Check sheet for the modelled part. Datum: model origin and axes. Units: mm. Face numbers are marked on the shaded views. A direction names the side the tool comes from. Give positions to 0.01 mm unless a question says otherwise; leave off trailing zeros. Write each loop counter-clockwise with the first axis right and the second up, starting at its lowest first coordinate (ties: lowest second). Pieces come first, ordered by that corner, then holes.
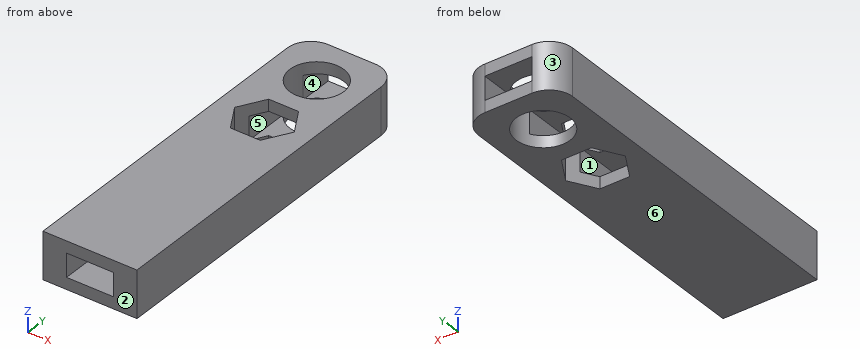
from build123d import *

# Parameters (mm, degrees)
ESQUISSE1_W                  = 40
ESQUISSE1_H                  = 20
BOSS_EXTRU_2_DEPTH           = 150
ESQUISSE2_R                  = 11.5
ENL_V_MAT_EXTRU_1_DEPTH      = 157.524758425
ENL_V_MAT_EXTRU_2_DEPTH      = 157.524758425
ENL_V_MAT_EXTRU_3_DEPTH      = 157.524758425
ENL_V_MAT_EXTRU_3_DEPTH_BACK = 157.524758425
ESQUISSE4_W                  = 20
ESQUISSE4_H                  = 10
CONG_2_R                     = 10
CONG_5_R                     = 10


with BuildPart() as part:
    # Esquisse1 → Boss.-Extru.2 (new body)
    with BuildSketch(Plane(origin=(0, 0, 0), x_dir=(1, 0, 0), z_dir=(0, 1, 0))):
        with Locations((-20, 10)):
            Rectangle(ESQUISSE1_W, ESQUISSE1_H)
    extrude(amount=BOSS_EXTRU_2_DEPTH)

    # Esquisse2 → Enlèv. mat.-Extru.1 (cut, through all)
    with BuildSketch(Plane.XY):
        with Locations((-20, 130)):
            Circle(ESQUISSE2_R)
    extrude(amount=-ENL_V_MAT_EXTRU_1_DEPTH, mode=Mode.SUBTRACT)

    # Esquisse3 → Enlèv. mat.-Extru.2 (cut, through all)
    with BuildSketch(Plane.XY):
        Polygon((-26.350852961, 111), (-32.701705922, 100), (-26.350852961, 89), (-13.649147039, 89), (-7.298294078, 100), (-13.649147039, 111), align=None)
    extrude(amount=-ENL_V_MAT_EXTRU_2_DEPTH, mode=Mode.SUBTRACT)

    # Esquisse4 → Enlèv. mat.-Extru.3 (cut, two sides: drawn at the far end of the back side and taken through both)
    with BuildSketch(Plane(origin=(0, 150, 0), x_dir=(1, 0, 0), z_dir=(0, 1, 0)).offset(-ENL_V_MAT_EXTRU_3_DEPTH_BACK)):
        with Locations((-20, 10)):
            Rectangle(ESQUISSE4_W, ESQUISSE4_H)
    extrude(amount=ENL_V_MAT_EXTRU_3_DEPTH + ENL_V_MAT_EXTRU_3_DEPTH_BACK, mode=Mode.SUBTRACT)

    # Congé2
    cong_2_edges = [part.edges().sort_by_distance(p)[0] for p in [
        (0, 150, -10),
    ]]
    fillet(cong_2_edges, radius=CONG_2_R - 0.0001)  # a hair under: the kernel refuses the full size

    # Congé5
    cong_5_edges = [part.edges().sort_by_distance(p)[0] for p in [
        (-40, 150, -10),
    ]]
    fillet(cong_5_edges, radius=CONG_5_R - 0.0001)  # a hair under: the kernel refuses the full size


solid = part.part
1) Gauge pin test, flat ends, axial feed: pin 1 (4.5 mm diameter, centred on x = -18.5, y = 141, fed in from +Z); pin 2 (1 mm diameter, centred on x = -22, z = -14, fed in from -Y). Record the tip position at first contact, or that the pin passes through.
2) Scan lines: L1, parallel to Y at x = -20, z = -15.75; L2, parallel to X at y = 85, z = -13.5; L3, parallel to X at y = 100, z = -12.5. Record each from-to range of solid material in increasing order.
3) Sectioned sample at A-A on y = 130. Record the boundary of the cut face in (x, z), then the cut area to 3 significant figures.
4) Sectioned sample at D-D on z = -2.25. Record the boundary of the cut face in (x, y), then the cut area to 3 significant figures.
5) Access from +Z, -Z, +X, -X, +Y, -Y to the whole of each face (thin tool, end or side, straight path). Record for the marked faces 5 and 6.
6) Sectioned sample at C-C on x = -20. Record the boundary of the cut face in (y, z), then the cut area to 3 significant figures.
7) Draft check along X on the marked faces 1, 2, 3 and 4. Enter one of: +X half, -X half, draft (parallel to the pull), parting line (faces both ways), or undercut.
Answers below:
1. pin 1: stops at z = 0
1. pin 2: passes through
2. L1: y = 0 to 89, 111 to 118.5, 141.5 to 150
2. L2: x = -40 to -30, -10 to 0
2. L3: x = -40 to -32.7, -7.3 to 0
3. outline: (-40, -20) - (-31.5, -20) - (-31.5, 0) - (-40, 0) - close; (-8.5, -20) - (0, -20) - (0, 0) - (-8.5, 0) - close
3. area: 340 mm2
4. outline: (-40, 0) - (0, 0) - (0, 140) arc R10 ccw to (-10, 150) - (-30, 150) arc R10 ccw to (-40, 140) - close; hole (-32.7, 100) - (-26.35, 89) - (-13.65, 89) - (-7.3, 100) - (-13.65, 111) - (-26.35, 111) - close; hole circle Ø23 at (-20, 130)
4. area: 5,120 mm2
5. face 5: +Y, -Y
5. face 6: -Z, +X, -X, +Y, -Y
6. outline: (0, -20) - (89, -20) - (89, -15) - (0, -15) - close; (0, -5) - (89, -5) - (89, 0) - (0, 0) - close; (111, -20) - (118.5, -20) - (118.5, -15) - (111, -15) - close; (111, -5) - (118.5, -5) - (118.5, 0) - (111, 0) - close; (141.5, -20) - (150, -20) - (150, -15) - (141.5, -15) - close; (141.5, -5) - (150, -5) - (150, 0) - (141.5, 0) - close
6. area: 1,050 mm2
7. face 1: undercut
7. face 2: draft
7. face 3: -X half
7. face 4: undercut
